Check sheet for the drawn part. Datum: minimum x, y, z corner. Units: mm. Coordinates: 2 decimals unless noted, no trailing zeros. Order: outer loops, then holes, each group sorted by start corner. A loop starts at its lowest first (then second) coordinate and runs counter-clockwise, first axis right, second up. Notation, with made-up numbers: M -31,-5 L -8,-5 A29 cw -8,27 Z; hole C 66,7.5 d10. An arc over 180 degrees is marked long. Answer in a Markdown table with one row per item. Add a question column.
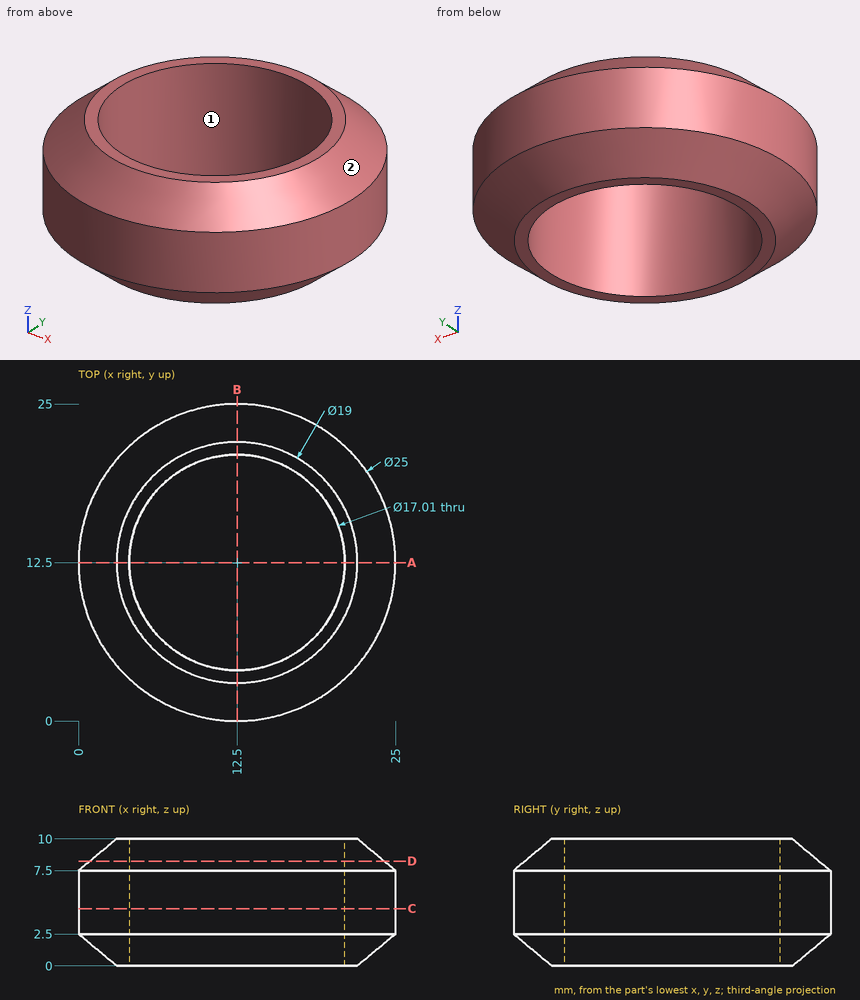
1. Section check C-C on z = 4.5. Enter the section's corners in (x, y) (3 decimals).
2. Go/stop test with flat-tipped pins: pin 1 Ø5 at (x, z) = (11.5, 8.5) entering from -Y; pin 2 Ø3 at (x, z) = (16, 8.5) entering from -Y; pin 3 Ø2 at (y, z) = (8.5, 4) entering from +X; pin 4 Ø5 at (x, z) = (19, 4) entering from +Y. Record where each tip stops, or that it passes through.
3. Scan lines: line 1 (Y direction, x = 12.5, z = 5.5) (3 decimals); line 2 (X direction, y = 12.5, z = 7.75) (3 decimals); line 3 (X direction, y = 8, z = 2). Record each from-to range of solid material in increasing order.
4. Section check D-D on z = 8.25. Enter the section's corners in (x, y) (3 decimals), then the cut area to 3 significant figures.
5. Release check for a two-part mould opening along X. For the marked faces 1 and 2 record: released by +X, released by -X, zero draft, split by the parting line, or undercut.
6. Section check A-A on y = 12.5. Enter the section's corners in (x, z) (3 decimals), then the cut area to 3 significant figures.
Result sheet:
| question | item | result |
|---|---|---|
| 1 | outline | C 12.5,12.5 d25; hole C 12.5,12.5 d17.01 |
| 2 | pin 1 | y = 0 |
| 2 | pin 2 | y = 0.23 |
| 2 | pin 3 | x = 24.63 |
| 2 | pin 4 | y = 24.34 |
| 3 | line 1 | 0 to 3.995, 21.005 to 25 |
| 3 | line 2 | 0.3 to 3.995, 21.005 to 24.7 |
| 3 | line 3 | 1.48 to 5.28, 19.72 to 23.52 |
| 4 | outline | C 12.5,12.5 d23.2; hole C 12.5,12.5 d17.01 |
| 4 | area | 195 mm^2 |
| 5 | face 1 | undercut |
| 5 | face 2 | split by the parting line |
| 6 | outline | M 0,2.5 L 3,0 L 3.995,0 L 3.995,10 L 3,10 L 0,7.5 Z; M 21.005,0 L 22,0 L 25,2.5 L 25,7.5 L 22,10 L 21.005,10 Z |
| 6 | area | 64.9 mm^2 |
